Autodesk Inventor part; units mm, degrees
ref_plane "YZ Plane" through (0, 0, 0) normal (1, 0, 0) x (0, 1, 0)
ref_plane "XZ Plane" through (0, 0, 0) normal (0, 1, 0) x (-1, 0, 0)
ref_plane "XY Plane" through (0, 0, 0) normal (0, 0, 1) x (1, 0, 0)
sketch "Sketch1" plane through (0, 0, 0) normal (0, 0, 1) x (1, 0, 0)
  circle A0 centre (0, 0) radius 1.4224
  circle A1 centre (0, 0) radius 3.175
  line L0 (0, 0) -> (-15.875, 0) construction
  circle A2 centre (-2.0016, -10.9307) radius 3.175
  circle A3 centre (-2.0016, -10.9307) radius 5 construction
  circle A4 centre (-2.0016, -10.9307) radius 1.5
  line L1 (0, 0) -> (-2.0016, -10.9307) construction
  line L2 (-2.0016, -10.9307) -> (-3.4771, -10.6606) construction
  line L3 (0, 0) -> (-2.0016, -10.9307) construction
  arc A5 (-5.0684, -10.109) -> (1.0652, -11.7525) centre (-2.0016, -10.9307) ccw
  arc A6 (-1.2212, -2.9308) -> (-15.875, 0) centre (-15.875, -38.1) ccw
  arc A7 (-15.875, 3.175) -> (-15.875, 0) centre (-15.875, 1.5875) ccw
  line L4 (-15.875, 3.175) -> (0, 3.175)
  line L5 (-2.0016, -10.9307) -> (-4.9305, 0) construction
  line L6 (1.0652, -10.109) -> (-1.8637, 0.8218)
  line L7 (-7.9973, -0.8218) -> (-5.0684, -11.7525)
  arc A8 (-5.0684, -11.7525) -> (1.0652, -10.109) centre (-2.0016, -10.9307) ccw
  arc A9 (-1.8637, 0.8218) -> (-7.9973, -0.8218) centre (-4.9305, 0) ccw
  circle A10 centre (6.7469, -0.7937) radius 3.175
  circle A11 centre (6.7469, -0.7937) radius 1.5
  line L8 (7.1178, 2.3595) -> (0.371, 3.1533)
  arc A12 (4.6726, -3.1975) -> (-0.0011, -6.1296) centre (2.7869, -5.3826) ccw
  circle A13 centre (6.7469, -0.7937) radius 5 construction
  point P0 (-5.0684, -10.109)
  point P1 (0, 3.175)
  point P2 (-7.9969, -0.8234)
  point P3 (1.0652, -10.109)
  point P4 (-0.8218, -3.0668)
  point P5 (-2.4653, 2.0008)
  point P6 (0.6312, -3.1116)
  point P7 (1.4598, -2.8195)
  point P8 (-1.4243, -1.0642)
  point P9 (-1.7024, 0.5129)
  point P10 (1.0652, -10.109)
  point P11 (-5.0684, -11.7525)
  dimension "d24" = 3
  dimension "d0" = 2.8448
  dimension "d1" = 6.35
  dimension "d9" = 15.875
  dimension "d22" = 6.35
  dimension "d23" = 10
  dimension "Arm_Length" = 11.1125
  dimension "d29" = 3.175
  dimension "d30" = 6.35
  dimension "d31" = 6.35
  dimension "d32" = 3
  dimension "d36" = 10
  dimension "Arm_Angle" = 105
  dimension "d38" = 4.7625
  dimension "d39" = 6.7469
  dimension "d40" = 0.7937
extrude "Extrusion1" add sketch "Sketch1" along normal blind 3.175
fillet "Fillet1" radius 3.175 1 edges at (-7.9969, -0.8234, 1.5875)
properties part number "Lever" material "Aluminum 6061"
Source: CAD feature listing. Evaluate the final solid. Frame: model axes, mm. A direction names the side the tool comes from. Round coordinates to 2 decimals unless told otherwise and drop trailing zeros. Loops run counter-clockwise (first coordinate to the right, second up) from the corner with the lowest first, then second, coordinate; pieces in that order, holes last.
(1) Section query C-C (x = -2.5). Output: boundary loops of the cut face in (y, z) (3 decimals).
From the geometry:
outline: (-14.066, 0) - (-12.345, 0) - (-12.345, 3.175) - (-14.066, 3.175) - close; (-9.516, 0) - (3.175, 0) - (3.175, 3.175) - (-9.516, 3.175) - close
(2) Section query B-B (z = 2.05). Give the number of separate pieces and of enclosed holes in the cut face, and give its area (3 significant figures).
From the geometry:
separate pieces: 1
enclosed holes: 3
area: 185 mm2
(3) Section query D-D (y = -8). Output: boundary loops of the cut face in (x, z) (3 decimals).
From the geometry:
outline: (-6.074, 0) - (0.5, 0) - (0.5, 3.175) - (-6.074, 3.175) - close
(4) Contact query for flat-ended pins moving along their axis: pin 1 Ø8 at (x, y) = (5, -8) entering from -Z; pin 2 Ø1 at (x, z) = (6.5, 1) entering from -Y. Output: stop coordinate, or through.
From the geometry:
pin 1: passes through
pin 2: stops at y = -3.97
(5) Access query for faces 1 (the flat face through (0.54, -8.15, 1.57)), 2 (the cylindrical face through (9.685, -1.996, 1.565)). Directions: +Z, -Z, +X, -X, +Y, -Y. A direction counts if a zero-diameter tool reaches every point of the face in a straight line with its end or side. Return the directions, or none.
From the geometry:
face 1: +Z, -Z, +X
face 2: +Z, -Z
(6) Pull-direction query (X, two-part tool) for faces 3 (the cylindrical face through (8.18, -1.24, 1.57)), 4 (the cylindrical face through (-1.11, -13.98, 1.57)), 5 (the cylindrical face through (-13, -0.11, 1.57)); classes: +X half, -X half, draft (parallel to the pull), parting line (faces both ways), or undercut.
From the geometry:
face 3: undercut
face 4: parting line
face 5: -X half
(7) Material intervals for probe 1 along X at (y, z) = (0.5, 0.5); probe 2 along X at (y, z) = (-3.25, 0.8); probe 3 along Y at (x, z) = (7.25, 2.1), sorted ascending.
From the geometry:
probe 1: x = -17.03 to -1.33, 1.33 to 5.99, 7.51 to 9.65
probe 2: x = -7.35 to 0.84, 4.74 to 8.76
probe 3: y = -3.93 to -2.21, 0.62 to 2.34
(8) Section query A-A (x = 7.5). Output: boundary loops of the cut face in (y, z) (3 decimals).
From the geometry:
outline: (-3.878, 0) - (-2.091, 0) - (-2.091, 3.175) - (-3.878, 3.175) - close; (0.504, 0) - (2.291, 0) - (2.291, 3.175) - (0.504, 3.175) - close
